Source: CAD feature listing. Evaluate the final solid. Frame: model axes, mm. A direction names the side the tool comes from. Give positions to 0.01 mm unless a question says otherwise; leave off trailing zeros. Return JSON: item names as keys, results as strings. Group by question number.
(1) Cut plane A-A on x = 0. Give the number of separate pieces and of enclosed holes in the cut face, then the cut area to 3 significant figures.
(2) Access query for faces 1 (the face through (-4.44, -6.11, 0.06)), 2 (the face through (0.715, -1.375, 6.023)). Directions: +Z, -Z, +X, -X, +Y, -Y. A direction counts if a zero-diameter tool reaches every point of the face in a straight line with its end or side. Return the directions, or none.
(3) Pin query (flat end, axial travel): pin 1 (4 mm diameter, centred on x = -4.5, z = -5.5, fed in from -Y); pin 2 (8 mm diameter, centred on y = -4, z = 2, fed in from -X); pin 3 (5 mm diameter, centred on x = 0, y = 0, fed in from -Z); pin 4 (2 mm diameter, centred on y = -4.5, z = 1.5, fed in from -X). Return the tip coordinate at first contact, or that it passes through.
(4) Ray query, line 1 (Z direction, x = -3.25, y = 1.75); line 2 (Y direction, x = 0, z = 5.55); line 3 (Y direction, x = -18, z = 1). Return the intervals inside material, ascending. Write a range as from..to.
(5) Draft query along Z for faces 3 (the face through (-3, 0, -4.1)), 4 (the face through (4.822, 1.323, -6.023)), 5 (the face through (-8, -4, -8)). Return one class per face: released by +Z, released by -Z, zero draft, split by the parting line, or undercut.
```python
from build123d import *

# Parameters (mm, degrees)
SKETCH1_R           = 1.55
BOSS_EXTRUDE1_DEPTH = 8
CUT_EXTRUDE1_DEPTH  = 4.1
CHAMFER1_START      = -4.1
CHAMFER1_DEPTH      = 8.2


with BuildPart() as part:
    # Sketch1 → Boss-Extrude1 (new, symmetric)
    with BuildSketch(Plane.XY):
        with BuildLine():
            Line((-20, -14), (-8, -14))
            add(Edge.make_bspline(
                [(1.429165494, -4.791397081), (-8, -7.603904107), (-8, -14)],
                knots=[0, 0, 0, 1, 1, 1], degree=2))
            ThreePointArc((1.429165494, -4.791397081), (4.791397081, 1.429165494), (-1.429165494, 4.791397081))
            add(Edge.make_bspline(
                [(-1.429165494, 4.791397081), (-20, -0.747863266), (-20, -14)],
                knots=[0, 0, 0, 1, 1, 1], degree=2))
        make_face()
        Circle(SKETCH1_R, mode=Mode.SUBTRACT)
    extrude(amount=BOSS_EXTRUDE1_DEPTH, both=True)

    # Sketch2 → Cut-Extrude1 (cut, symmetric)
    with BuildSketch(Plane.XY):
        with BuildLine():
            Line((-4.097628997, -7.253626281), (-7.078971892, 2.741575612))
            add(Edge.make_bspline(
                [(-1.429165494, 4.791397081), (-4.509542465, 3.872590228), (-7.078971892, 2.741575612)],
                knots=[0, 0, 0, 1, 1, 1], degree=2))
            ThreePointArc((-1.429165494, 4.791397081), (4.791397081, 1.429165494), (1.429165494, -4.791397081))
            add(Edge.make_bspline(
                [(-4.097628997, -7.253626281), (-1.934020936, -5.794559606), (1.429165494, -4.791397081)],
                knots=[0, 0, 0, 1, 1, 1], degree=2))
        make_face()
    extrude(amount=CUT_EXTRUDE1_DEPTH, both=True, mode=Mode.SUBTRACT)

    # Chamfer1: read off the stored shape, not the designer's step
    # Chamfer1 outline → Chamfer1 (cut)
    with BuildSketch(Plane.XY.offset(CHAMFER1_START)):
        with BuildLine():
            Line((-10.578223544, 0.965390038), (-4.792307112, -4.924659687))
            Line((-4.792307112, -4.924659687), (-7.078971892, 2.741575612))
            add(Edge.make_bspline(
                [(-7.078971892, 2.741575612), (-8.966458483, 1.910739435), (-10.578223544, 0.965390038)],
                knots=[0.165871758, 0.165871758, 0.165871758, 0.287720102, 0.287720102, 0.287720102], degree=2))
        make_face()
    extrude(amount=CHAMFER1_DEPTH, mode=Mode.SUBTRACT)


solid = part.part
```
Answers:
{
 "1": {"separate pieces": "4", "enclosed holes": "0", "area": "55.8 mm²"},
 "2": {"face 1": "+X, +Y", "face 2": "+Z, -Z"},
 "3": {"pin 1": "y = -9.47", "pin 2": "x = -18.9", "pin 3": "z = -8", "pin 4": "x = -17.62"},
 "4": {"line 1": "-8..-4.1, 4.1..8", "line 2": "-5.26..-1.55, 1.55..5", "line 3": "-14..-6.13"},
 "5": {"face 3": "undercut", "face 4": "zero draft", "face 5": "released by -Z"}
}
